Work out the finished part from the listing and answer in its coordinate system (mm). Face numbers are marked on the shaded views. A direction names the side the tool comes from. Round coordinates to 2 decimals unless told otherwise and drop trailing zeros. Write each loop counter-clockwise with the first axis right and the second up, starting at its lowest first coordinate (ties: lowest second). Pieces come first, ordered by that corner, then holes.
1. Determine the mould class of the marked faces 1, 2 and 3 for opening direction Z: pulls with the +Z half, pulls with the -Z half, needs draft (parallel to the pull), parting line crosses it, or undercut.
2. Straight lines are drawn through the part: probe 1 along Z at (x, y) = (74.5, 9); probe 2 along Y at (x, z) = (75.25, 7.25) (3 decimals); probe 3 along Y at (x, z) = (78, 2.25). For each, find the intervals that lie inside material, in ascending order.
3. Find section A-A (z = 9). Write down the section's boundary in (x, y) (3 decimals), and give its area (3 significant figures).
4. A flat-ended cylindrical pin translates along its axis: pin 1 Ø1 at (x, y) = (74, 5.5) entering from +Z. Find the tip coordinate at first contact, or state that the pin passes through.
5. Find section C-C (y = 0.75). Write down the section's boundary in (x, z).
6. Find section B-B (x = 75). Write down the section's boundary in (y, z) (3 decimals), and give its area (3 significant figures).
7. Find section D-D (x = 72.25). Write down the section's boundary in (y, z) (3 decimals), and give its area (3 significant figures).
8. A tool of negligible diameter and unlimited length cuts with its end or side. For the marked faces 4, 5 and 6, from which of +Z, -Z, +X, -X, +Y, -Y can it reach the whole face along a straight path? Write none if from no direction.
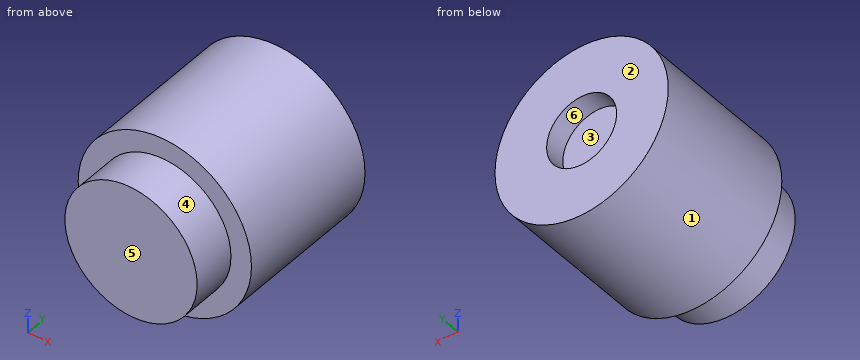
```python
from build123d import *

# Parameters (mm, degrees)
SKETCH015_R             = 4.8006
PAD008_DEPTH            = 3.175
SKETCH016_R             = 6.2865
PAD009_DEPTH            = 10.668
SKETCH017_R             = 2.54
POCKET006_DEPTH         = 1.524
BODY002_PLACEMENT_ANGLE = 90


with BuildPart() as part:
    # Sketch015 → Pad008 (new body)
    with BuildSketch(Plane.XY):
        Circle(SKETCH015_R)
    extrude(amount=PAD008_DEPTH)

    # Sketch016 (on Face2 of Pad008) → Pad009 (join)
    with BuildSketch(Plane(origin=(0, 0, 0), x_dir=(1, 0, 0), z_dir=(0, 0, -1))):
        Circle(SKETCH016_R)
    extrude(amount=PAD009_DEPTH)

    # Sketch017 (on Face3 of Pad009) → Pocket006 (cut)
    with BuildSketch(Plane(origin=(0, 0, -10.668), x_dir=(1, 0, 0), z_dir=(0, 0, -1))):
        Circle(SKETCH017_R)
    extrude(amount=-POCKET006_DEPTH, mode=Mode.SUBTRACT)


with BuildPart() as part_1:
    # Body002 placement: moved
    add(part.part.moved(Location((74.609706, 0, 5.728716))).rotate(Axis((74.609706, 0, 5.728716), (1, 0, 0)), BODY002_PLACEMENT_ANGLE))


solid = part_1.part
```
Worked answers:
1. face 1: parting line crosses it
1. face 2: needs draft
1. face 3: undercut
2. probe 1: z = -0.56 to 12.01
2. probe 2: y = -3.175 to 9.144
2. probe 3: y = 0 to 10.67
3. outline: (69.241, 0) - (71.096, 0) - (71.096, -3.175) - (78.123, -3.175) - (78.123, 0) - (79.978, 0) - (79.978, 10.668) - (69.241, 10.668) - close
3. area: 137 mm2
4. pin 1: stops at z = 12.01
5. outline: circle Ø12.57 at (74.61, 5.73)
6. outline: (-3.175, 0.944) - (0, 0.944) - (0, -0.546) - (10.668, -0.546) - (10.668, 3.219) - (9.144, 3.219) - (9.144, 8.239) - (10.668, 8.239) - (10.668, 12.003) - (0, 12.003) - (0, 10.513) - (-3.175, 10.513) - close
6. area: 157 mm2
7. outline: (-3.175, 1.548) - (0, 1.548) - (0, -0.098) - (10.668, -0.098) - (10.668, 4.789) - (9.144, 4.789) - (9.144, 6.669) - (10.668, 6.669) - (10.668, 11.556) - (0, 11.556) - (0, 9.909) - (-3.175, 9.909) - close
7. area: 148 mm2
8. face 4: -Y
8. face 5: +Z, -Z, +X, -X, -Y
8. face 6: +Y
